from build123d import *

# Parameters (mm, degrees)
CYLINDER037_R             = 2
CYLINDER037_DEPTH         = 10
BOX005_W                  = 37
BOX005_H                  = 4.5
BOX005_DEPTH              = 1.5
BOX006_W                  = 17
BOX006_H                  = 4.5
BOX006_DEPTH              = 1.5
BOX006_PLACEMENT_ANGLE    = 90
FUSION006_PITCH_ANGLE     = 90
FUSION006_PLACEMENT_ANGLE = -90


with BuildPart() as cylinder037:
    # Cylinder037 → Cylinder037 (new body)
    with BuildSketch(Plane(origin=(34.5, 34.5, 10.7594), x_dir=(1, 0, 0), z_dir=(0, 0, 1))):
        Circle(CYLINDER037_R)
    extrude(amount=CYLINDER037_DEPTH)


with BuildPart() as box005:
    # Box005 → Box005 (new body)
    with BuildSketch(Plane.XY):
        with Locations((18.5, 2.25)):
            Rectangle(BOX005_W, BOX005_H)
    extrude(amount=BOX005_DEPTH)


with BuildPart() as fusion006:
    # Box006 → Box006 (new body)
    with BuildSketch(Plane.XY):
        with Locations((8.5, 2.25)):
            Rectangle(BOX006_W, BOX006_H)
    extrude(amount=BOX006_DEPTH)


with BuildPart() as fusion006_1:
    # Box006 placement: moved
    add(fusion006.part.moved(Location((20.2342, -6.49055, 0))).rotate(Axis((20.2342, -6.49055, 0), (0, 0, 1)), BOX006_PLACEMENT_ANGLE))

    # Fusion004: union Box005
    add(box005.part)


with BuildPart() as fusion006_2:
    # Fusion004 placement: moved
    add(fusion006_1.part.moved(Location((16.4876, 32.0839, 17.56))))

    # Fusion006: union Cylinder037
    add(cylinder037.part)


with BuildPart() as fusion006_3:
    # Fusion006 pitch: moved
    add(fusion006_2.part.rotate(Axis((0, 0, 0), (0, 1, 0)), FUSION006_PITCH_ANGLE))


with BuildPart() as fusion006_4:
    # Fusion006 placement: moved
    add(fusion006_3.part.moved(Location((-48.6, 17.44, 105.53))).rotate(Axis((-48.6, 17.44, 105.53), (0, 0, 1)), FUSION006_PLACEMENT_ANGLE))


solid = fusion006_4.part
CAD build for the part. Positions are in the model's coordinates, mm. A direction names the side the tool comes from. Coordinates: 2 decimals unless noted, no trailing zeros. Loops run counter-clockwise (first coordinate to the right, second up) from the corner with the lowest first, then second, coordinate; pieces in that order, holes last. Notation, with made-up numbers: (73, 24.25) - (92, 24.25) arc R14 ccw to (92, 41.25) - close; hole circle Ø9 at (14, 25). An arc over 180 degrees is marked (long way). Write item = value, one per line. Start each with the question number.
Q1. Cut at C-C, the plane y = 2.75. List the corners of the cut face in (x, z).
Q2. Pull direction X, two halves, no side cores. Call faces 6 (the flat face through (-23.007, -1, 71)), 7 (the flat face through (-16.3, -0.12, 70.8)), 8 (the flat face through (-12.016, -1, 81)): pulls with the +X half, pulls with the -X half, needs draft (parallel to the pull), parting line crosses it, or undercut.
Q3. Cut at A-A, the plane x = -14.1. List the corners of the cut face in (y, z), then the cut area to 3 significant figures.
Q4. Drill centre lines: L1, parallel to Y at x = -15.5, z = 62.5; L2, parallel to Z at x = -12.75, y = 4.75; L3, parallel to X at y = 0.75, z = 70.5. Where is each one in solid material? Low to high.
Q5. Which spindle directions (+Z, -Z, +X, -X, +Y, -Y) get a long thin tool onto all of the face, cutting with end or side? Do faces 1 (the cylindrical face through (-13.499, -2.458, 69.122)), 2 (the flat face through (-16.516, -1, 81)), 3 (the flat face through (-9, -1, 73.308)), 4 (the flat face through (-12.016, -1, 61)), 5 (the flat face through (-16.516, -1, 61)). Say none if no direction does.
Q6. Cut at D-D, the plane z = 78.5. List the corners of the cut face in (x, y).
Q7. Cut at B-B, the plane z = 72. List the corners of the cut face in (x, y).
Q8. Flat gauge pins, fed straight in: pin 1 Ø2 at (x, z) = (-13, 66) entering from -Y; pin 2 Ø5 at (x, z) = (-18, 62) entering from +Y; pin 3 Ø0.8 at (x, y) = (-20, -1) entering from -Z; pin 4 Ø3 at (x, y) = (-18, 3) entering from +Z. Where does each tip first touch, or does it go through?
Computed:
q1.outline = circle Ø4 at (-14.1, 71.03)
q2.face_6 = pulls with the -X half
q2.face_7 = needs draft
q2.face_8 = pulls with the +X half
q3.outline = (-3.32, 69.03) - (-1.62, 69.03) - (-1.62, 52.04) - (-0.12, 52.04) - (-0.12, 69.03) - (6.68, 69.03) - (6.68, 73.03) - (-0.12, 73.03) - (-0.12, 89.04) - (-1.62, 89.04) - (-1.62, 73.03) - (-3.32, 73.03) - close
q3.area = 89.5 mm²
q4.L1 = -1.62 to -0.12
q4.L2 = 69.55 to 72.51
q4.L3 = -16.03 to -12.17
q5.face_1 = -Y
q5.face_2 = +Z, -X, +Y, -Y
q5.face_3 = +Z, +X, +Y, -Y
q5.face_4 = -Z, +X, +Y, -Y
q5.face_5 = -Z, -X, +Y, -Y
q6.outline = (-16.52, -1.62) - (-12.02, -1.62) - (-12.02, -0.12) - (-16.52, -0.12) - close
q7.outline = (-23.01, -1.62) - (-15.85, -1.62) - (-15.85, -3.32) - (-12.35, -3.32) - (-12.35, -1.62) - (-6.01, -1.62) - (-6.01, -0.12) - (-12.35, -0.12) - (-12.35, 6.68) - (-15.85, 6.68) - (-15.85, -0.12) - (-23.01, -0.12) - close
q8.pin_1 = -1.62
q8.pin_2 = -0.12
q8.pin_3 = 68.81
q8.pin_4 = through
